Design review of the part built by this model. Coordinates are the model's own, in mm. Face numbers are marked on the shaded views. A direction names the side the tool comes from. Give positions to 0.01 mm unless a question says otherwise; leave off trailing zeros. Loops run counter-clockwise (first coordinate to the right, second up) from the corner with the lowest first, then second, coordinate; pieces in that order, holes last. Notation, with made-up numbers: (27.5, 88) -> (41.5, 88) arc R22 ccw to (41.5, 126) -> close; hole circle Ø4 at (30.25, 46.5). An arc over 180 degrees is marked (long way). Answer in a Markdown table with one row per item. Add a question column.
(1) Consider section A-A on x = 0. Write out the cut boundary in (y, z) (3 decimals).
(2) For line 1 (Z direction, x = 0, y = -1.5) (3 decimals); line 2 (Z direction, x = 0.5, y = -6.75); line 3 (Y direction, x = -5.5, z = 4), list the stretches that pass through material, from the lowest coordinate up.
(3) For pin 1 (6 mm diameter, centred on x = 3, z = 2.5, fed in from -Y); pin 2 (2 mm diameter, centred on x = 0.5, y = -6, fed in from +Z); pin 3 (4.5 mm diameter, centred on x = 3, z = 0, fed in from +Y), all flat-tipped, find the tip position at first contact; note any pin that passes through.
(4) For the marked faces 5, 6 and 7, list the 3-axis set-ups (+Z, -Z, +X, -X, +Y, -Y) from which the entire face can be reached by the end or side of a thin tool; tool diameter is ignored.
(5) Draft analysis for pull direction Z (two halves, no side actions). For the marked faces 1, 2, 3 and 4, state which applies: +Z half, -Z half, draft (parallel to the pull), parting line (faces both ways), or undercut.
(6) Consider section B-B on y = -2. Write out the cut boundary in (x, z) (3 decimals).
(7) Consider section D-D on x = 3.75. Write out the cut boundary in (y, z).
(8) Consider section C-C on z = -1. Write out the cut boundary in (x, y) (3 decimals).
from build123d import *

# Parameters (mm, degrees)
F0_R     = 3.375
F1_DEPTH = 4
F2_W     = 14.75
F2_H     = 4
F3_DEPTH = 2
F4_R     = 3


with BuildPart() as f1:
    # F0 (on Front) → F1 (new body)
    with BuildSketch(Plane.XZ):
        with BuildLine():
            Line((7.375, -15), (7.375, 0))
            ThreePointArc((7.375, 0), (0, -7.375), (-7.375, 0))
            Line((-7.375, 0), (-7.375, -15))
            Line((-7.375, -15), (7.375, -15))
        make_face()
        with BuildLine():
            ThreePointArc((-7.375, 0), (0, -7.375), (7.375, 0))
            ThreePointArc((7.375, 0), (0, 7.375), (-7.375, 0))
        make_face()
        Circle(F0_R, mode=Mode.SUBTRACT)
    extrude(amount=F1_DEPTH)

    # F2 (on face) → F3 (join)
    with BuildSketch(Plane(origin=(0, 0, -15), x_dir=(1, 0, 0), z_dir=(0, 0, -1))):
        with Locations((0, -2)):
            Rectangle(F2_W, F2_H)
        with Locations((0, 2)):
            Rectangle(F2_W, F2_H)
        with Locations((0, 6)):
            Rectangle(F2_W, F2_H)
    extrude(amount=-F3_DEPTH)

    # F4
    f4_edges = [f1.edges().sort_by_distance(p)[0] for p in [
        (-7.375, -8, -14),
        (7.375, -8, -14),
        (-7.375, 4, -14),
        (7.375, 4, -14),
    ]]
    fillet(f4_edges, radius=F4_R)


solid = f1.part
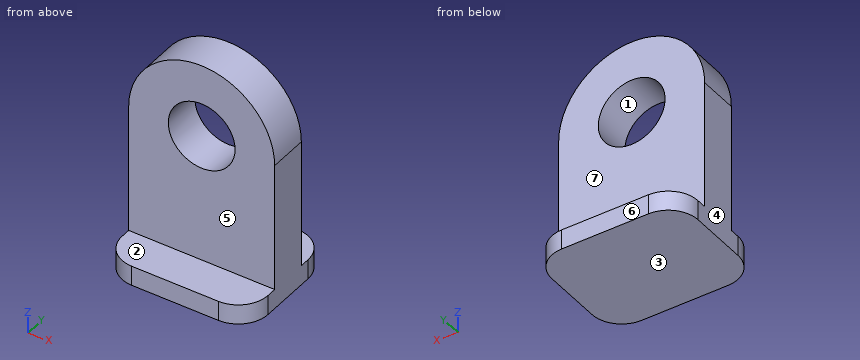
Values follow:
| question | item | result |
|---|---|---|
| 1 | outline | (-8, -15) -> (4, -15) -> (4, -13) -> (0, -13) -> (0, -3.375) -> (-4, -3.375) -> (-4, -13) -> (-8, -13) -> close; (-4, 3.375) -> (0, 3.375) -> (0, 7.375) -> (-4, 7.375) -> close |
| 2 | line 1 | -15 to -3.375, 3.375 to 7.375 |
| 2 | line 2 | -15 to -13 |
| 2 | line 3 | -4 to 0 |
| 3 | pin 1 | y = -4 |
| 3 | pin 2 | z = -13 |
| 3 | pin 3 | y = 0 |
| 4 | face 5 | +Z, +X, -X, -Y |
| 4 | face 6 | +Z, -Z, +X, -X, +Y |
| 4 | face 7 | +Z, +X, -X, +Y |
| 5 | face 1 | undercut |
| 5 | face 2 | +Z half |
| 5 | face 3 | -Z half |
| 5 | face 4 | draft |
| 6 | outline | (-7.375, -15) -> (7.375, -15) -> (7.375, 0) arc R7.375 ccw to (-7.375, 0) -> close; hole circle Ø6.75 at (0, 0) |
| 7 | outline | (-8, -15) -> (4, -15) -> (4, -13) -> (0, -13) -> (0, 6.35) -> (-4, 6.35) -> (-4, -13) -> (-8, -13) -> close |
| 8 | outline | (-7.375, -4) -> (-3.223, -4) -> (-3.223, 0) -> (-7.375, 0) -> close; (3.223, -4) -> (7.375, -4) -> (7.375, 0) -> (3.223, 0) -> close |
